```python
from build123d import *

# Parameters (mm, degrees)
SKETCH2_R           = 12.5
CUT_EXTRUDE1_DEPTH  = 2
BOSS_EXTRUDE1_DEPTH = 1.5
CIRPATTERN1_COUNT   = 6


with BuildPart() as part:
    # Sketch1 → Revolve1 (revolve)
    with BuildSketch(Plane(origin=(0, 0, 0), x_dir=(0, 0, -1), z_dir=(1, 0, 0))):
        Polygon((-45, 11), (-15, 11), (-15, -11), (-18, -11), (-18, 7), (-45, 7), (-55, 7), (-55, -11), (-58, -11), (-58, 11), align=None)
    revolve(axis=Axis((0, 42.640170011, 0), (0, -1, 0)))

    # Sketch2 → Cut-Extrude1 (cut)
    with BuildSketch(Plane(origin=(0, 11, 0), x_dir=(1, 0, 0), z_dir=(0, 1, 0))):
        with Locations(Location((0, 45, 0), (0, 0, 270))):
            Circle(SKETCH2_R)
        with Locations(Location((26.450336353, 36.405764747, 0), (0, 0, 270))):
            Circle(SKETCH2_R)
        with Locations(Location((42.797543233, 13.905764747, 0), (0, 0, 270))):
            Circle(SKETCH2_R)
        with Locations(Location((42.797543233, -13.905764747, 0), (0, 0, 270))):
            Circle(SKETCH2_R)
        with Locations(Location((26.450336353, -36.405764747, 0), (0, 0, 270))):
            Circle(SKETCH2_R)
        with Locations(Location((0, -45, 0), (0, 0, 270))):
            Circle(SKETCH2_R)
        with Locations(Location((-26.450336353, -36.405764747, 0), (0, 0, 270))):
            Circle(SKETCH2_R)
        with Locations(Location((-42.797543233, -13.905764747, 0), (0, 0, 270))):
            Circle(SKETCH2_R)
        with Locations(Location((-42.797543233, 13.905764747, 0), (0, 0, 270))):
            Circle(SKETCH2_R)
        with Locations(Location((-26.450336353, 36.405764747, 0), (0, 0, 270))):
            Circle(SKETCH2_R)
    extrude(amount=-CUT_EXTRUDE1_DEPTH, mode=Mode.SUBTRACT)

    # Sketch3 → Boss-Extrude1 (add, symmetric)
    with BuildSketch(Plane(origin=(0, 0, 0), x_dir=(0, 0, -1), z_dir=(1, 0, 0))):
        Polygon((-16.62069533, -11), (-16.62069533, 9), (-31.62069533, 9), align=None)
    boss_extrude1 = extrude(amount=BOSS_EXTRUDE1_DEPTH, both=True)

    # CirPattern1: Boss-Extrude1 ×6 about axis
    cirpattern1_axis = Axis((0, 0, 0), (0, 1, 0))
    for i in range(1, CIRPATTERN1_COUNT):
        add(boss_extrude1.rotate(cirpattern1_axis, i * 360 / CIRPATTERN1_COUNT))


solid = part.part
```
Here's how the part is built. I have some questions about the finished solid (model axes, mm). A direction names the side the tool comes from. Coordinates: 2 decimals unless noted, no trailing zeros. Order: outer loops, then holes, each group sorted by start corner. A loop starts at its lowest first (then second) coordinate and runs counter-clockwise, first axis right, second up.
Item 1: Thinking about a two-plate mould opening in X: for faces 1 (the face through (51.46, 0.15, 26.76)), 2 (the face through (21, -11, -51)), 3 (the face through (-34.056, 10.014, -46.325)), which applies, pulls with the +X half, pulls with the -X half, needs draft (parallel to the pull), parting line crosses it, or undercut?
Response values:
face 1: parting line crosses it
face 2: needs draft
face 3: undercut
Item 2: If we section it at B-B, the plane y = -0.75: List the corners of the cut face in (x, z) for me, then the cut area to 3 significant figures.
Response values:
outline: circle Ø116 at (0, 0); (-21.8, -10.86) - (-20.3, -13.45) - (-14.78, -10.27) arc R18 ccw to (-1.5, -17.94) - (-1.5, -24.31) - (1.5, -24.31) - (1.5, -17.94) arc R18 ccw to (14.78, -10.27) - (20.3, -13.45) - (21.8, -10.86) - (16.28, -7.67) arc R18 ccw to (16.28, 7.67) - (21.8, 10.86) - (20.3, 13.45) - (14.78, 10.27) arc R18 ccw to (1.5, 17.94) - (1.5, 24.31) - (-1.5, 24.31) - (-1.5, 17.94) arc R18 ccw to (-14.78, 10.27) - (-20.3, 13.45) - (-21.8, 10.86) - (-16.28, 7.67) arc R18 ccw to (-16.28, -7.67) - close; hole circle Ø110 at (0, 0); hole circle Ø30 at (0, 0)
area: 1,490 mm2
Item 3: I'm going to push flat-ended pins straight in: pin 1 Ø5 at (y, z) = (-2, -24.5) entering from +X; pin 2 Ø7.5 at (x, z) = (27.5, -32) entering from +Y; pin 3 Ø9.5 at (y, z) = (3, 22) entering from -X. Where does each tip first touch, or does it pass through?
Response values:
pin 1: stops at x = 53.67
pin 2: stops at y = 9
pin 3: stops at x = -55.38
Item 4: Which directions (+Z, -Z, +X, -X, +Y, -Y) give clear straight access to the entire face, cutting with the end or side of a thin tool? Please do faces 4 (the face through (30.2, 10.01, 48.33)), 5 (the face through (19.289, 2.601, -9.404)).
Response values:
face 4: +Y
face 5: -Y
Item 5: If we section it at C-C, the plane x = -3: List the corners of the cut face in (y, z) for me, then the cut area to 3 significant figures.
Response values:
outline: (-11, -57.92) - (11, -57.92) - (11, -57.13) - (9, -57.13) - (9, -32.87) - (11, -32.87) - (11, -14.7) - (-11, -14.7) - (-11, -17.75) - (7, -17.75) - (7, -54.92) - (-11, -54.92) - close; (-11, 14.7) - (11, 14.7) - (11, 32.87) - (9, 32.87) - (9, 57.13) - (11, 57.13) - (11, 57.92) - (-11, 57.92) - (-11, 54.92) - (7, 54.92) - (7, 17.75) - (-11, 17.75) - close
area: 467 mm2
Item 6: I need wall thicknesses on probe 1 along Z at (x, y) = (7.5, 0.5); probe 2 along X at (y, z) = (6.75, 0); probe 3 along X at (y, z) = (-6, 16). Which ranges of each line are inside material? Lowest first, please.
Response values:
probe 1: z = -57.51 to -54.49, -16.36 to -12.99, 12.99 to 16.36, 54.49 to 57.51
probe 2: x = -58 to -55, -18 to -15, 15 to 18, 55 to 58
probe 3: x = -55.75 to -52.62, -8.25 to 8.25, 52.62 to 55.75
Item 7: If we section it at D-D, the plane x = 33.5: List the corners of the cut face in (y, z) for me, then the cut area to 3 significant figures.
Response values:
outline: (-11, -47.35) - (11, -47.35) - (11, -46.73) - (9, -46.73) - (9, -26.08) - (11, -26.08) - (11, -22.26) - (9, -22.26) - (9, -5.55) - (11, -5.55) - (11, 5.55) - (9, 5.55) - (9, 22.26) - (11, 22.26) - (11, 26.08) - (9, 26.08) - (9, 46.73) - (11, 46.73) - (11, 47.35) - (-11, 47.35) - (-11, 43.62) - (7, 43.62) - (7, -43.62) - (-11, -43.62) - close
area: 364 mm2
Item 8: If we section it at A-A, the plane z = 0: List the corners of the cut face in (x, y) for me, then the cut area to 3 significant figures.
Response values:
outline: (-58, -11) - (-55, -11) - (-55, 7) - (-18, 7) - (-18, -11) - (-15, -11) - (-15, 11) - (-58, 11) - close; (15, -11) - (18, -11) - (18, 7) - (55, 7) - (55, -11) - (58, -11) - (58, 11) - (15, 11) - close
area: 560 mm2
